from build123d import *

# Parameters (mm, degrees)
ESQUISSE1_W             = 80
ESQUISSE1_H             = 63
BOSS_EXTRU_1_DEPTH      = 1.5
ESQUISSE2_R             = 1.25
ESQUISSE2_R_2           = 2
ESQUISSE2_W             = 55
ESQUISSE2_H             = 17
ENL_V_MAT_EXTRU_1_DEPTH = 75.640806534
CONG_1_R                = 4


with BuildPart() as part:
    # Esquisse1 → Boss.-Extru.1 (new body)
    with BuildSketch(Plane(origin=(0, 0, 0), x_dir=(1, 0, 0), z_dir=(0, 1, 0))):
        with Locations((0, -31.5)):
            Rectangle(ESQUISSE1_W, ESQUISSE1_H)
    extrude(amount=BOSS_EXTRU_1_DEPTH)

    # Esquisse2 → Enlèv. mat.-Extru.1 (cut, through all)
    with BuildSketch(Plane(origin=(0, 1.5, 0), x_dir=(1, 0, 0), z_dir=(0, 1, 0))):
        with Locations(Location((-37.5, -44, 0), (0, 0, 270))):
            Circle(ESQUISSE2_R)
        with Locations(Location((-37.5, -9, 0), (0, 0, 270))):
            Circle(ESQUISSE2_R)
        with Locations(Location((-25, -9, 0), (0, 0, 270))):
            Circle(ESQUISSE2_R_2)
        with Locations(Location((25, -9, 0), (0, 0, 90))):
            Circle(ESQUISSE2_R_2)
        with Locations(Location((37.5, -9, 0), (0, 0, 90))):
            Circle(ESQUISSE2_R)
        with Locations(Location((37.5, -44, 0), (0, 0, 90))):
            Circle(ESQUISSE2_R)
        with Locations((0, -54.5)):
            Rectangle(ESQUISSE2_W, ESQUISSE2_H)
    extrude(amount=-ENL_V_MAT_EXTRU_1_DEPTH, mode=Mode.SUBTRACT)

    # Congé1
    cong_1_edges = [part.edges().sort_by_distance(p)[0] for p in [
        (-27.5, 0.75, 63),
        (-27.5, 0.75, 46),
        (27.5, 0.75, 46),
        (27.5, 0.75, 63),
        (-40, 0.75, 0),
        (40, 0.75, 0),
        (40, 0.75, 63),
        (-40, 0.75, 63),
    ]]
    fillet(cong_1_edges, radius=CONG_1_R)


solid = part.part
Here's how the part is built. I have some questions about the finished solid (model axes, mm). A direction names the side the tool comes from. Coordinates: 2 decimals unless noted, no trailing zeros. Loops run counter-clockwise (first coordinate to the right, second up) from the corner with the lowest first, then second, coordinate; pieces in that order, holes last.
1. If we mould it in two halves opening along X, with no side actions, what happens to faces 3 (the cylindrical face through (-38.26, 0.76, 8.01)), 4 (the flat face through (-1, 0, 24)), 5 (the cylindrical face through (-38.859, 0.76, 1.203))? For each: pulls with the +X half, pulls with the -X half, needs draft (parallel to the pull), parting line crosses it, or undercut.
2. Imagine slicing it at C-C, the plane z = 44. Please give me the cut outline in (x, y), and give its area (4 significant figures).
3. For P1, Ø6.5, axis at x = -25, z = 9, coming from the +Y side, with a flat end and sliding along its axis, tell me the tip position at first contact or that it passes through.
4. Imagine slicing it at A-A, the plane z = 9. Please give me the cut outline in (x, y), and give its area (4 significant figures).
5. For faces 1 (the cylindrical face through (38.26, 0.76, 44.99)), 2 (the cylindrical face through (28.703, 0.74, 61.859)), which set-ups out of +Z, -Z, +X, -X, +Y, -Y let a thin tool reach every point of the face, with its end or its side?
6. Imagine slicing it at B-B, the plane y = 1.1. Please give me the cut outline in (x, z), and give its area (3 significant figures).
7. Imagine slicing it at D-D, the plane x = 25. Please give me the cut outline in (y, z).
8. I need wall thicknesses on L1, parallel to X at y = 1.1, z = 9; L2, parallel to X at y = 0.55, z = 44; L3, parallel to Z at x = -15, y = 0.9. Which ranges of each line are inside material? Lowest first, please.
Taken from the geometry:
1. face 3: undercut
1. face 4: needs draft
1. face 5: pulls with the -X half
2. outline: (-40, 0) - (-38.75, 0) - (-38.75, 1.5) - (-40, 1.5) - close; (-36.25, 0) - (36.25, 0) - (36.25, 1.5) - (-36.25, 1.5) - close; (38.75, 0) - (40, 0) - (40, 1.5) - (38.75, 1.5) - close
2. area: 112.5 mm2
3. P1: stops at y = 1.5
4. outline: (-40, 0) - (-38.75, 0) - (-38.75, 1.5) - (-40, 1.5) - close; (-36.25, 0) - (-27, 0) - (-27, 1.5) - (-36.25, 1.5) - close; (-23, 0) - (23, 0) - (23, 1.5) - (-23, 1.5) - close; (27, 0) - (36.25, 0) - (36.25, 1.5) - (27, 1.5) - close; (38.75, 0) - (40, 0) - (40, 1.5) - (38.75, 1.5) - close
4. area: 100.5 mm2
5. face 1: +Y, -Y
5. face 2: +Z, +Y, -Y
6. outline: (-40, 4) arc R4 ccw to (-36, 0) - (36, 0) arc R4 ccw to (40, 4) - (40, 59) arc R4 ccw to (36, 63) - (31.5, 63) arc R4 ccw to (27.5, 59) - (27.5, 50) arc R4 cw to (23.5, 46) - (-23.5, 46) arc R4 cw to (-27.5, 50) - (-27.5, 59) arc R4 ccw to (-31.5, 63) - (-36, 63) arc R4 ccw to (-40, 59) - close; hole circle Ø2.5 at (-37.5, 9); hole circle Ø2.5 at (-37.5, 44); hole circle Ø4 at (-25, 9); hole circle Ø4 at (25, 9); hole circle Ø2.5 at (37.5, 9); hole circle Ø2.5 at (37.5, 44)
6. area: 4,050 mm2
7. outline: (0, 0) - (1.5, 0) - (1.5, 7) - (0, 7) - close; (0, 11) - (1.5, 11) - (1.5, 46.29) - (0, 46.29) - close
8. L1: x = -40 to -38.75, -36.25 to -27, -23 to 23, 27 to 36.25, 38.75 to 40
8. L2: x = -40 to -38.75, -36.25 to 36.25, 38.75 to 40
8. L3: z = 0 to 46
